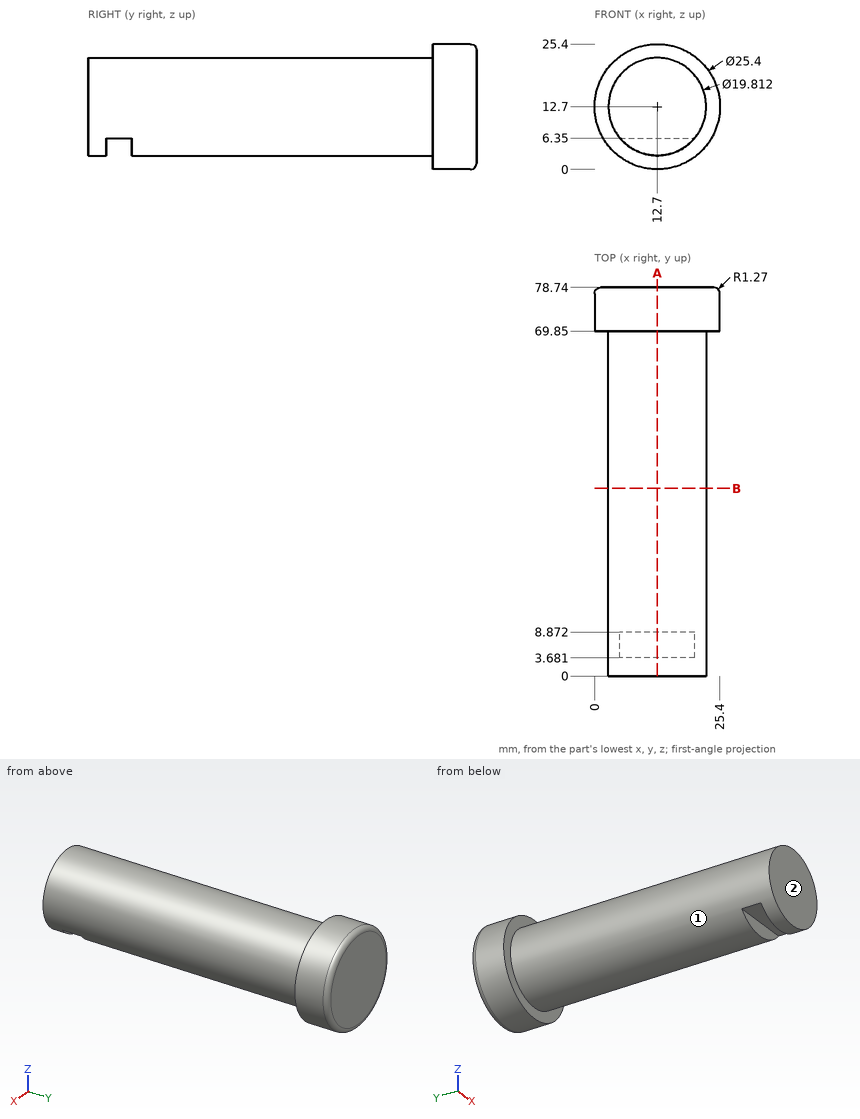
Could you check a few things on this drawing? It's one solid part, dimensions in mm from its lowest x, y, z. A direction names the side the tool comes from. Round coordinates to 2 decimals unless told otherwise and drop trailing zeros. Order: outer loops, then holes, each group sorted by start corner. A loop starts at its lowest first (then second) coordinate and runs counter-clockwise, first axis right, second up. Notation, with made-up numbers: M -28,45 L -10,45 A6 ccw -10,54 Z; hole C 16,42 d4. An arc over 180 degrees is marked long. Return JSON: item names as keys, results as strings. Group by question number.
1. I'm going to push flat-ended pins straight in: pin 1 Ø5 at (y, z) = (12, 20) entering from -X (1 decimal); pin 2 Ø3 at (x, z) = (14, 5) entering from -Y; pin 3 Ø10 at (x, y) = (10.5, 48) entering from +Z; pin 4 Ø10 at (y, z) = (28.5, 16.5) entering from -X. Where does each tip first touch, or does it pass through?
2. If we section it at B-B on y = 38: List the corners of the cut face in (x, z) for me, then the cut area to 3 significant figures.
3. If we section it at A-A on x = 12.7: List the corners of the cut face in (y, z) for me.
4. On a 3-axis mill with a long thin cutter (end or side, diameter ignored), from which of +Z, -Z, +X, -X, +Y, -Y can I reach the whole of each face in a straight line? I mean the marked faces 1 and 2. Say none if no direction works.
5. Please list where these lines run through material, in increasing order: probe 1 along Y at (x, z) = (21.5, 7.75); probe 2 along X at (y, z) = (14.5, 12.75); probe 3 along X at (y, z) = (9, 6.5) (1 decimal).
Reply:
{
 "1": {"pin 1": "x = 4", "pin 2": "y = 0", "pin 3": "z = 22.61", "pin 4": "x = 2.79"},
 "2": {"outline": "C 12.7,12.7 d19.81", "area": "308 mm^2"},
 "3": {"outline": "M 0,2.79 L 3.68,2.79 L 3.68,6.35 L 8.87,6.35 L 8.87,2.79 L 69.85,2.79 L 69.85,0 L 77.47,0 A1.27 ccw 78.74,1.27 L 78.74,24.13 A1.27 ccw 77.47,25.4 L 69.85,25.4 L 69.85,22.61 L 0,22.61 Z"},
 "4": {"face 1": "-Y", "face 2": "+Z, -Z, +X, -X, -Y"},
 "5": {"probe 1": "69.85 to 78.74", "probe 2": "2.79 to 22.61", "probe 3": "5 to 20.4"}
}
